Can you work these out from the model? Positions are in its coordinate system, mm. A direction names the side the tool comes from. Coordinates: 2 decimals unless noted, no trailing zeros. Loops run counter-clockwise (first coordinate to the right, second up) from the corner with the lowest first, then second, coordinate; pieces in that order, holes last. Notation, with made-up numbers: M 63,-10.5 L 79,-10.5 A29 cw 79,27.5 Z; hole C 42.5,32.25 d3. An arc over 180 degrees is marked long. Answer as a JSON object with one key per item and string values. Group by question number.
Item 1: Which directions (+Z, -Z, +X, -X, +Y, -Y) give clear straight access to the entire face, cutting with the end or side of a thin tool? Please do faces 1 (the cylindrical face through (87.63, -57.97, 36.48)), 2 (the flat face through (100, -35.041, 37)).
Item 2: We'd pull the mould along X, two halves only. Please class faces 3 (the flat face through (100, -56, 40)), 4 (the flat face through (82.794, -50, 37)), 5 (the cylindrical face through (87.72, -45.5, 36.48)): +X half, -X half, draft (parallel to the pull), parting line (faces both ways), or undercut.
Item 3: I'm going to push flat-ended pins straight in: pin 1 Ø5 at (x, y) = (91, -58.5) entering from -Z; pin 2 Ø3 at (x, y) = (111.5, -59) entering from -Z. Where does each tip first touch, or does it pass through?
Item 4: Suppose I cut it at A-A (y = -52.5). Write out the boundary of the cut face in (x, z) (3 decimals).
Item 5: Suppose I cut it at C-C (z = 36.75). Write out the boundary of the cut face in (x, y), then the cut area to 3 significant figures.
Item 6: If I drill on line 1 (Y direction, x = 111, z = 36.8); line 2 (Y direction, x = 110, z = 35.5); line 3 (X direction, y = -49.75, z = 36.1), over which ranges is the centre line in solid material (lowest first)?
Item 7: Suppose I cut it at B-B (x = 102.5). Write out the boundary of the cut face in (y, z), then the cut area to 3 significant figures.
Item 8: Suppose I cut it at D-D (y = -62.25). Write out the boundary of the cut face in (x, z).
```python
from build123d import *

# Parameters (mm, degrees)
SKETCH032_W     = 35.340293
SKETCH032_H     = 29.690987
PAD011_DEPTH    = 5
SKETCH033_R     = 3.176208
POCKET014_DEPTH = 3
SKETCH034_R     = 7
POCKET015_DEPTH = 5


with BuildPart() as part:
    # Sketch032 → Pad011 (new body)
    with BuildSketch(Plane.XY):
        with Locations((100.463696, -49.886112)):
            Rectangle(SKETCH032_W, SKETCH032_H)
    extrude(amount=PAD011_DEPTH)

    # Sketch033 (on Face5 of Pad011) → Pocket014 (cut)
    with BuildSketch(Plane(origin=(0, 0, 0), x_dir=(1, 0, 0), z_dir=(0, 0, -1))):
        with Locations((90.151108, 59.905067)):
            Circle(SKETCH033_R)
        with Locations((90.236954, 47.436592)):
            Circle(SKETCH033_R)
        with Locations((111.203728, 59.926529)):
            Circle(SKETCH033_R)
        with Locations((111.203728, 47.500977)):
            Circle(SKETCH033_R)
    extrude(amount=-POCKET014_DEPTH, mode=Mode.SUBTRACT)

    # Sketch034 (on Face4 of Pocket014) → Pocket015 (cut)
    with BuildSketch(Plane(origin=(0, 0, 0), x_dir=(1, 0, 0), z_dir=(0, 0, -1))):
        with Locations((100.58239, 47.488678)):
            Circle(SKETCH034_R)
    extrude(amount=-POCKET015_DEPTH, mode=Mode.SUBTRACT)


with BuildPart() as part_1:
    # Body004 placement: moved
    add(part.part.moved(Location((0, 0, 35))))


solid = part_1.part
```
From the geometry:
{
 "1": {"face 1": "-Z", "face 2": "+Z, -Z, +X, -X, +Y"},
 "2": {"face 3": "draft", "face 4": "-X half", "face 5": "undercut"},
 "3": {"pin 1": "z = 35", "pin 2": "z = 38"},
 "4": {"outline": "M 82.794,35 L 95.695,35 L 95.695,40 L 82.794,40 Z; M 105.47,35 L 118.134,35 L 118.134,40 L 105.47,40 Z"},
 "5": {"outline": "M 82.79,-64.73 L 118.13,-64.73 L 118.13,-35.04 L 82.79,-35.04 Z; hole C 90.15,-59.91 d6.35; hole C 90.24,-47.44 d6.35; hole C 100.58,-47.49 d14; hole C 111.2,-59.93 d6.35; hole C 111.2,-47.5 d6.35", "area": "769 mm2"},
 "6": {"line 1": "-64.73 to -63.1, -56.76 to -50.67, -44.33 to -35.04", "line 2": "-64.73 to -62.87, -56.99 to -50.44, -44.56 to -35.04", "line 3": "82.79 to 88.06, 92.41 to 93.96, 107.21 to 108.96, 113.45 to 118.13"},
 "7": {"outline": "M -64.73,35 L -54.22,35 L -54.22,40 L -64.73,40 Z; M -40.76,35 L -35.04,35 L -35.04,40 L -40.76,40 Z", "area": "81.1 mm2"},
 "8": {"outline": "M 82.79,35 L 88.01,35 L 88.01,38 L 92.29,38 L 92.29,35 L 109.04,35 L 109.04,38 L 113.37,38 L 113.37,35 L 118.13,35 L 118.13,40 L 82.79,40 Z"}
}
